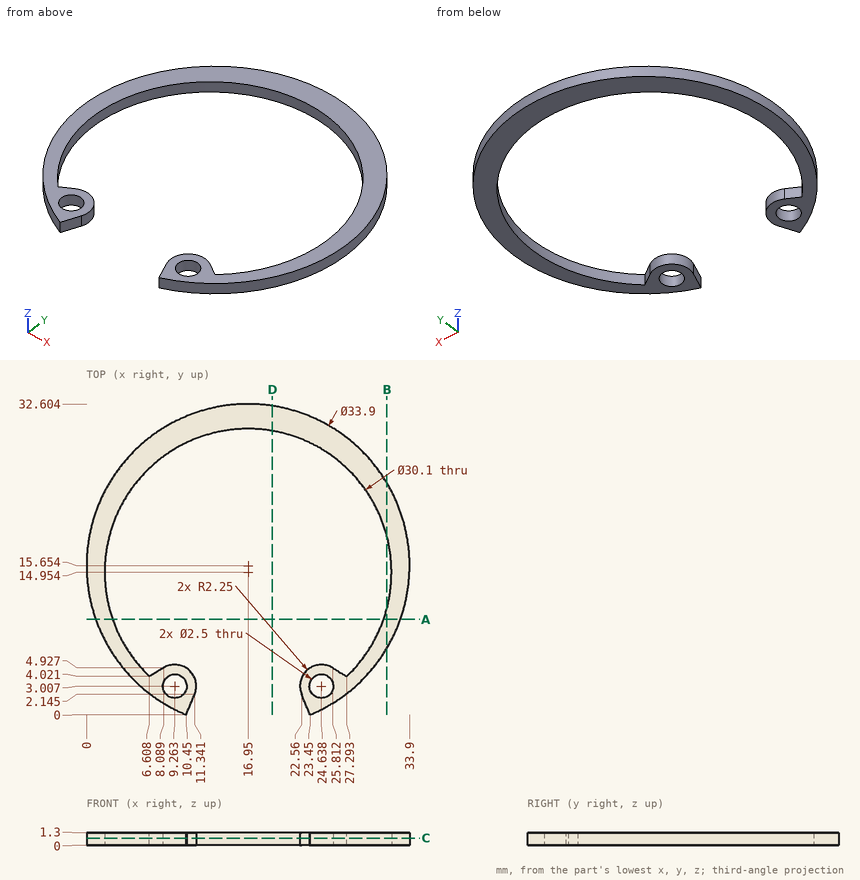
Answer from the drawing. Dimensions are ordinates in mm from the lowest x, y and z of the part. Coordinates: 2 decimals unless noted, no trailing zeros. Write each loop counter-clockwise with the first axis right and the second up, starting at its lowest first coordinate (ties: lowest second). Pieces come first, ordered by that corner, then holes. Notation, with made-up numbers: M 84.5,-27 L 119.5,-27 A28 ccw 119.5,-7 Z; hole C 16.5,-40 d6. An arc over 180 degrees is marked long. Write item = value, one per line.
1. The part is cut by section B-B (x = 31.5). Determine the outline of the cut face in (y, z), then the cut area to 3 significant figures.
Solution:
outline = M 6.96,0 L 11.11,0 L 11.11,1.3 L 6.96,1.3 Z; M 18.8,0 L 24.35,0 L 24.35,1.3 L 18.8,1.3 Z
area = 12.6 mm2
2. A flat-ended cylindrical pin translates along its axis: pin 1 (1.5 mm diameter, centred on x = 24, y = 6, fed in from -Z). Find the tip coordinate at first contact, or state that the pin passes through.
Solution:
pin_1 = through
3. Straight lines are drawn through the part: line 1 (X direction, y = 3, z = 0.1) (1 decimal); line 2 (Y direction, x = 17, z = 0.7) (1 decimal); line 3 (X direction, y = 8.5, z = 1.05) (1 decimal). For each, find the intervals that lie inside material, in ascending order. Write a range as from..to.
Solution:
line_1 = 5.7..8, 10.5..11.5, 22.4..23.4, 25.9..28.2
line_2 = 30..32.6
line_3 = 1.6..3.4, 30.5..32.3
4. The part is cut by section A-A (y = 10). Determine the outline of the cut face in (x, z).
Solution:
outline = M 0.97,0 L 2.74,0 L 2.74,1.3 L 0.97,1.3 Z; M 31.16,0 L 32.93,0 L 32.93,1.3 L 31.16,1.3 Z
5. The part is cut by section D-D (x = 19.5). Determine the outline of the cut face in (y, z).
Solution:
outline = M 29.79,0 L 32.41,0 L 32.41,1.3 L 29.79,1.3 Z
6. The part is cut by section C-C (z = 0.75). State how many separate pieces and enclosed holes the cut face has.
Solution:
separate_pieces = 1
enclosed_holes = 2
